Check sheet for the modelled part. Datum: model origin and axes. Units: mm. A direction names the side the tool comes from. Coordinates: 2 decimals unless noted, no trailing zeros. Loops run counter-clockwise (first coordinate to the right, second up) from the corner with the lowest first, then second, coordinate; pieces in that order, holes last.
```python
from build123d import *

# Parameters (mm, degrees)
F2_SIZE = 0.5
F3_R    = 1


with BuildPart() as f1:
    # F0 (on Right) → F1 (revolve)
    with BuildSketch(Plane.YZ):
        Polygon((0, 6), (0, 0), (23, 0), (23, 9), (11, 9), (11, 4.5), (9, 4.5), (9, 6), align=None)
    revolve(axis=Axis((0, 11.5, 0), (0, -1, 0)))

    # F2
    f2_edges = [f1.edges().sort_by_distance(p)[0] for p in [
        (0, 0, -6),
        (0, 9, -6),
    ]]
    chamfer(f2_edges, length=F2_SIZE)

    # F3
    f3_edges = [f1.edges().sort_by_distance(p)[0] for p in [
        (0, 11, -9),
        (0, 23, -9),
    ]]
    fillet(f3_edges, radius=F3_R)


solid = f1.part
```
1) Scan lines: line 1 (Y direction, x = 4.5, z = 2.25); line 2 (Y direction, x = 5.5, z = -1); line 3 (Z direction, x = -2, y = 12). Record each from-to range of solid material in increasing order.
Answer sheet:
line 1: y = 0 to 9, 11 to 23
line 2: y = 0.09 to 8.91, 11 to 23
line 3: z = -8.77 to 8.77
2) Depth check by flat-ended pin: pin 1 (2 mm diameter, centred on x = -5, z = 6, fed in from -Y); pin 2 (1.5 mm diameter, centred on y = 10.5, z = -1, fed in from -X); pin 3 (8 mm diameter, centred on y = 8.5, z = -2.5, fed in from -X). Enter the tip coordinate at first touch or a pass-through.
Answer sheet:
pin 1: stops at y = 11
pin 2: stops at x = -8.61
pin 3: stops at x = -8.99
3) Section check A-A on z = 0. Enter the section's corners in (x, y).
Answer sheet:
outline: (-9, 12) arc R1 ccw to (-8, 11) - (-4.5, 11) - (-4.5, 9) - (-5.5, 9) - (-6, 8.5) - (-6, 0.5) - (-5.5, 0) - (5.5, 0) - (6, 0.5) - (6, 8.5) - (5.5, 9) - (4.5, 9) - (4.5, 11) - (8, 11) arc R1 ccw to (9, 12) - (9, 22) arc R1 ccw to (8, 23) - (-8, 23) arc R1 ccw to (-9, 22) - close
4) Section check D-D on y = 10. Enter the section's corners in (x, z), plus the area to 3 significant figures.
Answer sheet:
outline: circle Ø9 at (0, 0)
area: 63.6 mm2
5) Set-up check for faces 4 (the cylindrical face through (-8.923, 16.93, -1.172)), 5 (the cylindrical face through (-4.46, 9.99, -0.59)): record each of +Z, -Z, +X, -X, +Y, -Y from which the full face is reachable in a straight line by a thin tool's end or side.
Answer sheet:
face 4: +Y, -Y
face 5: none
6) Section check C-C on y = 19. Enter the section's corners in (x, z), plus the area to 3 significant figures.
Answer sheet:
outline: circle Ø18 at (0, 0)
area: 254 mm2
7) Section check B-B on x = 0. Enter the section's corners in (y, z), plus the area to 3 significant figures.
Answer sheet:
outline: (0, -5.5) - (0.5, -6) - (8.5, -6) - (9, -5.5) - (9, -4.5) - (11, -4.5) - (11, -8) arc R1 ccw to (12, -9) - (22, -9) arc R1 ccw to (23, -8) - (23, 8) arc R1 ccw to (22, 9) - (12, 9) arc R1 ccw to (11, 8) - (11, 4.5) - (9, 4.5) - (9, 5.5) - (8.5, 6) - (0.5, 6) - (0, 5.5) - close
area: 341 mm2
8) Mould release check, pull along Y, two halves, no side actions. Record for faces 1 (the flat face through (3.4, 11, 3.4)), 2 (the flat face through (0, 23, 0)), 3 (the cylindrical face through (0, 4, -6)): +Y half, -Y half, draft (parallel to the pull), parting line (faces both ways), or undercut.
Answer sheet:
face 1: undercut
face 2: +Y half
face 3: draft
